```python
from build123d import *

# Parameters (mm, degrees)
F0_W     = 170
F0_H     = 35
F1_DEPTH = 3
F2_D     = 2
F2_DEPTH = 40
F3_D     = 2
F3_DEPTH = 40
F5_D     = 2
F5_DEPTH = 40


with BuildPart() as f1:
    # F0 (on Front) → F1 (new body)
    with BuildSketch(Plane.XZ):
        Polygon((37, 35), (37, 53), (-37, 53), (-37, -53), (37, -53), (37, -35), (37, 0), align=None)
        with Locations((122, -17.5)):
            Rectangle(F0_W, F0_H)
        with Locations((122, 17.5)):
            Rectangle(F0_W, F0_H)
    extrude(amount=F1_DEPTH)

    # F2
    with Locations(Plane(origin=(0, 0, 0), x_dir=(1, 0, 0), z_dir=(0, 1, 0))):
        with Locations((-29, 0), (29, 0)):
            Hole(F2_D / 2, depth=F2_DEPTH)

    # F3
    with Locations(Plane(origin=(0, 0, 0), x_dir=(1, 0, 0), z_dir=(0, 1, 0))):
        with Locations((29, -30), (-29, -30), (29, 30), (-29, 30)):
            Hole(F3_D / 2, depth=F3_DEPTH)

    # F5
    with Locations(Plane(origin=(0, 0, 0), x_dir=(1, 0, 0), z_dir=(0, 1, 0))):
        with Locations((0, -30), (0, 30), (200, -30), (200, 30)):
            Hole(F5_D / 2, depth=F5_DEPTH)


solid = f1.part
```
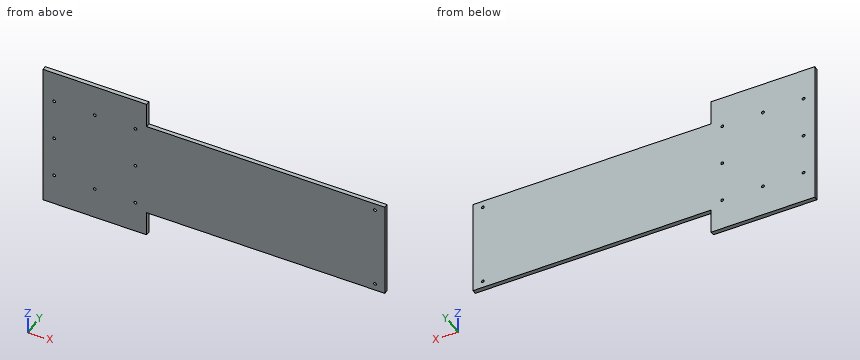
Geometry check sheet. Reference: the model listing, model coordinates, mm. Coordinates: 2 decimals unless noted, no trailing zeros. Order: outer loops, then holes, each group sorted by start corner. A loop starts at its lowest first (then second) coordinate and runs counter-clockwise, first axis right, second up. Notation, with made-up numbers: (87.25, -39.75) - (143.25, -39.75) arc R35 cw to (143.25, -6.75) - close; hole circle Ø4 at (54.25, 71). An arc over 180 degrees is marked (long way). Answer in a Markdown table with one row per item. Add a question column.
1. Gauge pin test, flat ends, axial feed: pin 1 Ø0.9 at (x, y) = (135, -1.5) entering from +Z; pin 2 Ø1.5 at (x, y) = (92.5, -2.5) entering from -Z; pin 3 Ø1.5 at (y, z) = (-2, -40) entering from +X; pin 4 Ø1.8 at (x, z) = (-29, -30) entering from +Y. Record the tip position at first contact, or that the pin passes through.
2. Material ranges on L1, parallel to Z at x = 29, y = -1.25; L2, parallel to X at y = -0.95, z = -30; L3, parallel to Z at x = 0, y = -1.4, recorded low to high. Write a range as [from, to].
3. Section check B-B (x = 80.5). Enter the section's corners in (y, z), plus the area to 3 significant figures.
4. Section check A-A (y = -1.4). Give the number of separate pieces and of enclosed holes in the cut face, plus the area to 3 significant figures.
Data:
| question | item | result |
|---|---|---|
| 1 | pin 1 | stops at z = 35 |
| 1 | pin 2 | stops at z = -35 |
| 1 | pin 3 | stops at x = 37 |
| 1 | pin 4 | passes through |
| 2 | L1 | z = [-53, -31], [-29, -1], [1, 29], [31, 53] |
| 2 | L2 | x = [-37, -30], [-28, -1], [1, 28], [30, 199], [201, 207] |
| 2 | L3 | z = [-53, -31], [-29, 29], [31, 53] |
| 3 | outline | (-3, -35) - (0, -35) - (0, 35) - (-3, 35) - close |
| 3 | area | 210 mm² |
| 4 | separate pieces | 1 |
| 4 | enclosed holes | 10 |
| 4 | area | 19,700 mm² |
